Verification items for the finished model (mm, model axes). A direction names the side the tool comes from. Give positions to 0.01 mm unless a question says otherwise; leave off trailing zeros. Write each loop counter-clockwise with the first axis right and the second up, starting at its lowest first coordinate (ties: lowest second). Pieces come first, ordered by that corner, then holes. Notation, with made-up numbers: (-21.5, 1) -> (-16.5, 1) arc R22 ccw to (-16.5, 7) -> close; hole circle Ø8 at (68, -19). An arc over 180 degrees is marked (long way). Use one line per item in the form item = value. Start each with the question number.
(1) Depth check by flat-ended pin: pin 1 Ø0.5 at (y, z) = (2, -36) entering from -X; pin 2 Ø0.8 at (y, z) = (1.5, -36) entering from +X; pin 3 Ø0.5 at (y, z) = (1, -42) entering from -X. Enter the tip coordinate at first touch or a pass-through.
(2) Scan lines: L1, parallel to X at y = 1.6, z = -33.1; L2, parallel to X at y = 1.8, z = -13; L3, parallel to Z at x = 30.5, y = 1.8. Record each from-to range of solid material in increasing order.
(3) Section check B-B, the plane x = -40. Record the cut outline in (y, z).
(4) Section check D-D, the plane y = 0.85. State how many separate pieces and enclosed holes the cut face has, plus the area to 3 significant figures.
(5) Section check A-A, the plane z = -33.1. Record the cut outline in (x, y).
(6) Release check for a two-part mould opening along Z. For faces 1 (the face through (17.85, 1.52, -20.99)), 2 (the face through (-11, 2, -8.125)), 3 (the face through (-15, 1, -12)) record: pulls with the +Z half, pulls with the -Z half, needs draft (parallel to the pull), parting line crosses it, or undercut.
(7) Section check C-C, the plane z = -21.5. Record the cut outline in (x, y), plus the area to 3 significant figures.
(8) Set-up check for faces 4 (the face through (-29, 1, -40.1)), 5 (the face through (46, 2, -26)), 6 (the face through (-7, 1, -24)): record each of +Z, -Z, +X, -X, +Y, -Y from which the full face is reachable in a straight line by a thin tool's end or side.
from build123d import *

# Parameters (mm, degrees)
SKETCH1_R           = 3.25
SKETCH1_W           = 14
SKETCH1_H           = 32.5
BOSS_EXTRUDE1_DEPTH = 3
FILLET1_R           = 10
FILLET2_R           = 1
FILLET3_R           = 5
CUT_EXTRUDE1_REACH  = 65.841
SKETCH2_W           = 4
SKETCH2_H           = 1


with BuildPart() as part:
    # Sketch1 → Boss-Extrude1 (new body)
    with BuildSketch(Plane(origin=(0, 0, 0), x_dir=(1, 0, 0), z_dir=(0, 1, 0))):
        Polygon((-47, 40.1), (-15, 40.1), (-15, 43.1), (15, 43.1), (15, 40.1), (47, 40.1), (47, 24), (15, 24), (15, 0), (-15, 0), (-15, 24), (-47, 24), align=None)
        with Locations(Location((40, 33.1, 0), (0, 0, 270))):
            Circle(SKETCH1_R, mode=Mode.SUBTRACT)
        with Locations(Location((-40, 33.1, 0), (0, 0, 90))):
            Circle(SKETCH1_R, mode=Mode.SUBTRACT)
        with Locations((0, 23.85)):
            Rectangle(SKETCH1_W, SKETCH1_H, mode=Mode.SUBTRACT)
    extrude(amount=BOSS_EXTRUDE1_DEPTH)

    # Fillet1
    fillet1_edges = [part.edges().sort_by_distance(p)[0] for p in [
        (-15, 1.5, -24),
        (15, 1.5, -24),
        (15, 1.5, 0),
        (-15, 1.5, 0),
    ]]
    fillet(fillet1_edges, radius=FILLET1_R)

    # Fillet2
    fillet2_edges = [part.edges().sort_by_distance(p)[0] for p in [
        (-15, 1.5, -40.1),
        (-15, 1.5, -43.1),
        (15, 1.5, -43.1),
        (15, 1.5, -40.1),
        (-7, 1.5, -40.1),
        (-7, 1.5, -7.6),
        (7, 1.5, -7.6),
        (7, 1.5, -40.1),
    ]]
    fillet(fillet2_edges, radius=FILLET2_R)

    # Fillet3
    fillet3_edges = [part.edges().sort_by_distance(p)[0] for p in [
        (-47, 1.5, -24),
        (-47, 1.5, -40.1),
        (47, 1.5, -40.1),
        (47, 1.5, -24),
    ]]
    fillet(fillet3_edges, radius=FILLET3_R)

    # Sketch2 → Cut-Extrude1 (cut, up to next)
    with BuildSketch(Plane(origin=(0, 3, 0), x_dir=(1, 0, 0), z_dir=(0, 1, 0)), mode=Mode.PRIVATE) as cut_extrude1_sk1:
        with Locations((10.6, 14.225)):
            Rectangle(SKETCH2_W, SKETCH2_H)
    cut_extrude1_tool1 = extrude(cut_extrude1_sk1.sketch, amount=-CUT_EXTRUDE1_REACH, mode=Mode.PRIVATE) & part.part
    # Sketch2 → Cut-Extrude1 (cut, up to next)
    with BuildSketch(Plane(origin=(0, 3, 0), x_dir=(1, 0, 0), z_dir=(0, 1, 0)), mode=Mode.PRIVATE) as cut_extrude1_sk2:
        with Locations((10.6, 41.8)):
            Rectangle(SKETCH2_W, SKETCH2_H)
    cut_extrude1_tool2 = extrude(cut_extrude1_sk2.sketch, amount=-CUT_EXTRUDE1_REACH, mode=Mode.PRIVATE) & part.part
    # Sketch2 → Cut-Extrude1 (cut, up to next)
    with BuildSketch(Plane(origin=(0, 3, 0), x_dir=(1, 0, 0), z_dir=(0, 1, 0)), mode=Mode.PRIVATE) as cut_extrude1_sk3:
        with Locations((-10.6, 41.8)):
            Rectangle(SKETCH2_W, SKETCH2_H)
    cut_extrude1_tool3 = extrude(cut_extrude1_sk3.sketch, amount=-CUT_EXTRUDE1_REACH, mode=Mode.PRIVATE) & part.part
    # Sketch2 → Cut-Extrude1 (cut, up to next)
    with BuildSketch(Plane(origin=(0, 3, 0), x_dir=(1, 0, 0), z_dir=(0, 1, 0)), mode=Mode.PRIVATE) as cut_extrude1_sk4:
        with Locations((-10.6, 36.15)):
            Rectangle(SKETCH2_W, SKETCH2_H)
    cut_extrude1_tool4 = extrude(cut_extrude1_sk4.sketch, amount=-CUT_EXTRUDE1_REACH, mode=Mode.PRIVATE) & part.part
    # Sketch2 → Cut-Extrude1 (cut, up to next)
    with BuildSketch(Plane(origin=(0, 3, 0), x_dir=(1, 0, 0), z_dir=(0, 1, 0)), mode=Mode.PRIVATE) as cut_extrude1_sk5:
        with Locations((10.6, 36.15)):
            Rectangle(SKETCH2_W, SKETCH2_H)
    cut_extrude1_tool5 = extrude(cut_extrude1_sk5.sketch, amount=-CUT_EXTRUDE1_REACH, mode=Mode.PRIVATE) & part.part
    # Sketch2 → Cut-Extrude1 (cut, up to next)
    with BuildSketch(Plane(origin=(0, 3, 0), x_dir=(1, 0, 0), z_dir=(0, 1, 0)), mode=Mode.PRIVATE) as cut_extrude1_sk6:
        with Locations((-10.6, 14.225)):
            Rectangle(SKETCH2_W, SKETCH2_H)
    cut_extrude1_tool6 = extrude(cut_extrude1_sk6.sketch, amount=-CUT_EXTRUDE1_REACH, mode=Mode.PRIVATE) & part.part
    # Sketch2 → Cut-Extrude1 (cut, up to next)
    with BuildSketch(Plane(origin=(0, 3, 0), x_dir=(1, 0, 0), z_dir=(0, 1, 0)), mode=Mode.PRIVATE) as cut_extrude1_sk7:
        with Locations((-10.6, 8.625)):
            Rectangle(SKETCH2_W, SKETCH2_H)
    cut_extrude1_tool7 = extrude(cut_extrude1_sk7.sketch, amount=-CUT_EXTRUDE1_REACH, mode=Mode.PRIVATE) & part.part
    # Sketch2 → Cut-Extrude1 (cut, up to next)
    with BuildSketch(Plane(origin=(0, 3, 0), x_dir=(1, 0, 0), z_dir=(0, 1, 0)), mode=Mode.PRIVATE) as cut_extrude1_sk8:
        with Locations((10.6, 8.625)):
            Rectangle(SKETCH2_W, SKETCH2_H)
    cut_extrude1_tool8 = extrude(cut_extrude1_sk8.sketch, amount=-CUT_EXTRUDE1_REACH, mode=Mode.PRIVATE) & part.part
    add(cut_extrude1_tool1.solids().sort_by_distance((10.6, 3, -14.225))[0], mode=Mode.SUBTRACT)
    add(cut_extrude1_tool2.solids().sort_by_distance((10.6, 3, -41.8))[0], mode=Mode.SUBTRACT)
    add(cut_extrude1_tool3.solids().sort_by_distance((-10.6, 3, -41.8))[0], mode=Mode.SUBTRACT)
    add(cut_extrude1_tool4.solids().sort_by_distance((-10.6, 3, -36.15))[0], mode=Mode.SUBTRACT)
    add(cut_extrude1_tool5.solids().sort_by_distance((10.6, 3, -36.15))[0], mode=Mode.SUBTRACT)
    add(cut_extrude1_tool6.solids().sort_by_distance((-10.6, 3, -14.225))[0], mode=Mode.SUBTRACT)
    add(cut_extrude1_tool7.solids().sort_by_distance((-10.6, 3, -8.625))[0], mode=Mode.SUBTRACT)
    add(cut_extrude1_tool8.solids().sort_by_distance((10.6, 3, -8.625))[0], mode=Mode.SUBTRACT)


solid = part.part
Completed:
q1.pin_1 = -46.96
q1.pin_2 = 46.97
q1.pin_3 = -15
q2.L1 = -47 to -43.25, -36.75 to -7, 7 to 36.75, 43.25 to 47
q2.L2 = -15 to -7, 7 to 15
q2.L3 = -40.1 to -24
q3.outline = (0, -40.1) -> (3, -40.1) -> (3, -36.35) -> (0, -36.35) -> close; (0, -29.85) -> (3, -29.85) -> (3, -24) -> (0, -24) -> close
q4.separate_pieces = 1
q4.enclosed_holes = 11
q4.area = 1,750 mm²
q5.outline = (-47, 0) -> (-43.25, 0) -> (-43.25, 3) -> (-47, 3) -> close; (-36.75, 0) -> (-7, 0) -> (-7, 3) -> (-36.75, 3) -> close; (7, 0) -> (36.75, 0) -> (36.75, 3) -> (7, 3) -> close; (43.25, 0) -> (47, 0) -> (47, 3) -> (43.25, 3) -> close
q6.face_1 = pulls with the +Z half
q6.face_2 = undercut
q6.face_3 = needs draft
q7.outline = (-18.39, 0) -> (-7, 0) -> (-7, 3) -> (-18.39, 3) -> close; (7, 0) -> (18.39, 0) -> (18.39, 3) -> (7, 3) -> close
q7.area = 68.3 mm²
q8.face_4 = -Z, -X, +Y, -Y
q8.face_5 = +Z, +X, +Y, -Y
q8.face_6 = +Y, -Y
